Design review of the part built by this model. Coordinates are the model's own, in mm. A direction names the side the tool comes from. Give positions to 0.01 mm unless a question says otherwise; leave off trailing zeros. Loops run counter-clockwise (first coordinate to the right, second up) from the corner with the lowest first, then second, coordinate; pieces in that order, holes last. Notation, with made-up numbers: (60.5, -7.75) -> (115.5, -7.75) arc R21 ccw to (115.5, 12.25) -> close; hole circle Ø11 at (35, -27). An arc over 180 degrees is marked (long way). Use a Markdown table: item, result. Add a question column.
1. Add section B-B (z = 6). State the section outline as (x, y) points.
2. Add section A-A (x = -61.5). State the section outline as (y, z) points.
3. Draft analysis for pull direction Z (two halves, no side actions). For faces 1 (the flat face through (-41.69, -0.23, 85.77)), 2 (the flat face through (-39, 0, 34.649)), 3 (the cylindrical face through (-73.285, -0.235, 64.273)), state which applies: pulls with the +Z half, pulls with the -Z half, needs draft (parallel to the pull), parting line crosses it, or undercut.
4. To check wall thickness, follow line 1 (X direction, y = -1, z = 66.5); line 2 (Z direction, x = -11.5, y = -6); line 3 (X direction, y = 5, z = 25). State the ranges of each line that lie inside material, in increasing order.
5. For pin 1 Ø4 at (y, z) = (-32, 50) entering from +X; pin 2 Ø19 at (x, y) = (2.5, -4.5) entering from +Z; pin 3 Ø2 at (x, z) = (19.5, 13) entering from +Y, all flat-tipped, find the tip position at first contact; note any pin that passes through.
6. For faces 4 (the cylindrical face through (-71.438, -0.057, 65.12)), 5 (the flat face through (0, 0, 3.048)), 6 (the flat face through (24, -22, 3.857)), list the 3-axis set-ups (+Z, -Z, +X, -X, +Y, -Y) from which the entire face can be reached by the end or side of a thin tool; tool diameter is ignored.
7. Add section C-C (z = 25). State the section outline as (x, y) points.
```python
from build123d import *

# Parameters (mm, degrees)
F0_R     = 33.02
F1_DEPTH = 78.232
F1_TAPER = -5.63
F3_R     = 34.036
F3_R_2   = 33.02
F4_DEPTH = 78.232
F4_TAPER = -5.63
F5_T     = -3.048
F9_W     = 2.032
F9_H     = 12.7


with BuildPart() as f1:
    # F0 (on Top) → F1 (new body)
    with BuildSketch(Plane.XY):
        Circle(F0_R)
    extrude(amount=F1_DEPTH, taper=F1_TAPER)

    # F3 (on face) → F4 (join)
    with BuildSketch(Plane(origin=(0, 0, 0), x_dir=(1, 0, 0), z_dir=(0, 0, -1))):
        Circle(F3_R)
        Circle(F3_R_2, mode=Mode.SUBTRACT)
    extrude(amount=-F4_DEPTH, taper=F4_TAPER)

    # F5
    f5_openings = [f1.faces().sort_by_distance(p)[0] for p in [
        (0, 0, 78.232),
    ]]
    offset(amount=F5_T, openings=f5_openings, kind=Kind.INTERSECTION)

    # F6 (on Front) → F7 (revolve, cut)
    with BuildSketch(Plane.XZ):
        with BuildLine():
            Line((32.6848506642, 3.2326551154), (32.3112107695, 0))
            Line((32.3112107695, 0), (44.0889932215, 0))
            Line((44.0889932215, 0), (44.0889932215, 54.3507039547))
            Line((44.0889932215, 54.3507039547), (39.4513271749, 54.3507039547))
            Line((39.4513271749, 54.3507039547), (39.3896299843, 54.2361003943))
            Line((39.3896299843, 54.2361003943), (36.3627001643, 23.5965643078))
            ThreePointArc((36.3627001643, 23.5965643078), (35.2832636057, 16.619062002), (33.4441874208, 9.8022797333))
            Line((33.4441874208, 9.8022797333), (32.8385867178, 4.5627476647))
            Line((32.8385867178, 4.5627476647), (32.7852428872, 4.1012278712))
            Line((32.7852428872, 4.1012278712), (32.7570124771, 3.8569842))
            Line((32.7570124771, 3.8569842), (32.0890299447, 3.8569842))
            Line((32.0890299447, 3.8569842), (32.0060770141, 3.2326551154))
            Line((32.0060770141, 3.2326551154), (32.6848506642, 3.2326551154))
        make_face()
    revolve(axis=Axis((0, 0, 38.8779193163), (0, 0, 1)), mode=Mode.SUBTRACT)

    # F2 (on Front) → F10 (revolve)
    with BuildSketch(Plane.XZ):
        Polygon((0, -3.6346768029), (0, 0), (-32.1533791721, 0), (-31.7057520151, -3.6346768029), align=None)
    revolve(axis=Axis((0, 0, -1.8173384015), (0, 0, 1)))

    # F11: sweep along a path in F8
    with BuildLine(Plane.XZ) as f11_path:
        Line((-38.7114321376, 73.8900886301), (-40.5326529346, 93.9235173966))
        ThreePointArc((-40.5326529346, 93.9235173966), (-43.168569243, 98.5178624573), (-48.3705692501, 99.5154882628))
        ThreePointArc((-48.3705692501, 99.5154882628), (-73.1825968463, 63.6219410958), (-40.5282266438, 34.6793159842))
        Line((-40.5282266438, 34.6793159842), (-35.0613184273, 34.6793159842))
    # F9 (on face) → F11 (sweep)
    with BuildSketch(Plane.XY.offset(78.232)):
        with Locations((-70.6608099122, -0.1456312999)):
            Rectangle(F9_W, F9_H)
    sweep(path=f11_path.line)


solid = f1.part
```
Taken from the geometry:
| question | item | result |
|---|---|---|
| 1 | outline | circle Ø66.01 at (0, 0); hole circle Ø63.13 at (0, 0) |
| 2 | outline | (-6.5, 42.19) -> (6.2, 42.19) -> (6.2, 44.73) -> (-6.5, 44.73) -> close; (-6.5, 90.41) -> (6.2, 90.41) -> (6.2, 92.95) -> (-6.5, 92.95) -> close |
| 3 | face 1 | undercut |
| 3 | face 2 | pulls with the -Z half |
| 3 | face 3 | parting line crosses it |
| 4 | line 1 | x = -73.43 to -71.52, -40.58 to -37.52, 37.52 to 40.58 |
| 4 | line 2 | z = -3.63 to 3.05 |
| 4 | line 3 | x = -36.16 to -33.06, 33.06 to 36.16 |
| 5 | pin 1 | stops at x = 24.88 |
| 5 | pin 2 | stops at z = 3.05 |
| 5 | pin 3 | stops at y = 29.09 |
| 6 | face 4 | +Y, -Y |
| 6 | face 5 | +Z |
| 6 | face 6 | none |
| 7 | outline | circle Ø73 at (0, 0); hole circle Ø66.88 at (0, 0) |
